from build123d import *

# Parameters (mm, degrees)
BOSS_EXTRUDE1_DEPTH = 4


with BuildPart() as part:
    # Sketch1 → Boss-Extrude1 (new body)
    with BuildSketch(Plane(origin=(0, 0, 0), x_dir=(0, 1, 0), z_dir=(0, 0, 1))):
        Polygon((0, 0), (136.832013798, -79), (213.480030045, 241), (53.636318593, 233.929787175), align=None)
        with BuildLine():
            Line((167.998036635, 192.356313097), (193.088330721, 186.346559132))
            ThreePointArc((193.088330721, 186.346559132), (194.64139794, 183.815159872), (192.10999868, 182.262092653))
            Line((192.10999868, 182.262092653), (167.019704595, 188.271846618))
            ThreePointArc((167.019704595, 188.271846618), (165.466637376, 190.803245878), (167.998036635, 192.356313097))
        make_face(mode=Mode.SUBTRACT)
        with BuildLine():
            Line((118.32403237, -15.029111125), (143.414326455, -21.03886509))
            ThreePointArc((143.414326455, -21.03886509), (145.945725715, -19.485797871), (144.392658496, -16.954398611))
            Line((144.392658496, -16.954398611), (119.30236441, -10.944644646))
            ThreePointArc((119.30236441, -10.944644646), (116.77096515, -12.497711865), (118.32403237, -15.029111125))
        make_face(mode=Mode.SUBTRACT)
    extrude(amount=BOSS_EXTRUDE1_DEPTH)


solid = part.part
The model under review builds one solid part; all positions refer to its coordinate system, in mm. A direction names the side the tool comes from. Give positions to 0.01 mm unless a question says otherwise; leave off trailing zeros. Loops run counter-clockwise (first coordinate to the right, second up) from the corner with the lowest first, then second, coordinate; pieces in that order, holes last. Notation, with made-up numbers: (1, 58) -> (60, 58) arc R11 ccw to (60, 65) -> close; hole circle Ø6 at (25, 85.5). An arc over 180 degrees is marked (long way). Answer as a JSON object with one key per item and string values. Group by question number.
Q1. Draft analysis for pull direction Y (two halves, no side actions). For faces 1 (the flat face through (-78.76, 174.62, 1.97)), 2 (the flat face through (13.99, 132.02, 1.97)), 3 (the flat face through (-83, 105, 0)), state which applies: pulls with the +Y half, pulls with the -Y half, needs draft (parallel to the pull), parting line crosses it, or undercut.
Q2. Take a section at A-A (z = 2.2). Write out the cut boundary in (x, y).
Q3. Take a section at C-C (y = 65). Write out the cut boundary in (x, z), plus the area to 3 significant figures.
Q4. Wall thickness on line 1 along X through (y, z) = (124, 0.9); line 2 along Y through (x, z) = (-211.5, 3.3); line 3 along Y through (x, z) = (-115, 2.3): over which ranges is each line inside the solid? List them lowest first.
Q5. Tool access review of faces 4 (the flat face through (-83, 105, 4)), 5 (the flat face through (-189.394, 180.368, 1.972)): name each direction out of +Z, -Z, +X, -X, +Y, -Y from which nothing blocks a thin tool from reaching the whole face with its end or side.
Q6. Insertion check: pin 1 (1 mm diameter, centred on x = -145, z = 2.5, fed in from +Y); pin 2 (1 mm diameter, centred on y = 32, z = 2.5, fed in from +X); pin 3 (1 mm diameter, centred on y = 22, z = 1, fed in from +X). Each pin has a flat end and moves straight along its axis. Give the tip position at first contact, or say it passes through.
Q7. Take a section at B-B (x = -137.5). Write out the cut boundary in (y, z).
Answer below:
{
 "1": {"face 1": "pulls with the +Y half", "face 2": "undercut", "face 3": "needs draft"},
 "2": {"outline": "(-241, 213.48) -> (-233.93, 53.64) -> (0, 0) -> (79, 136.83) -> close; hole (-192.36, 168) arc R2.1 ccw to (-188.27, 167.02) -> (-182.26, 192.11) arc R2.1 ccw to (-186.35, 193.09) -> close; hole (10.94, 119.3) arc R2.1 ccw to (15.03, 118.32) -> (21.04, 143.41) arc R2.1 ccw to (16.95, 144.39) -> close"},
 "3": {"outline": "(-234.43, 0) -> (37.53, 0) -> (37.53, 4) -> (-234.43, 4) -> close", "area": "1,090 mm2"},
 "4": {"line 1": "x = -237.04 to 12.07, 16.39 to 71.59", "line 2": "y = 48.49 to 206.41", "line 3": "y = 26.37 to 183.3"},
 "5": {"face 4": "+Z, +X, -X, +Y, -Y", "face 5": "+Z, -Z"},
 "6": {"pin 1": "stops at y = 190.61", "pin 2": "stops at x = 18.76", "pin 3": "stops at x = 12.99"},
 "7": {"outline": "(31.53, 0) -> (188.69, 0) -> (188.69, 4) -> (31.53, 4) -> close"}
}
